Geometry: final body of the model. Coordinates: model frame, mm. Face numbers are marked on the shaded views. A direction names the side the tool comes from. Round coordinates to 2 decimals unless told otherwise and drop trailing zeros. Write each loop counter-clockwise with the first axis right and the second up, starting at its lowest first coordinate (ties: lowest second). Pieces come first, ordered by that corner, then holes. Notation, with made-up numbers: (81, -37.75) -> (129, -37.75) arc R32 ccw to (129, 1.25) -> close; hole circle Ø4 at (-12.75, 67). An arc over 180 degrees is marked (long way). Use one line per item in the form item = value. Start each with the question number.
1. Cut plane B-B, the plane x = 0. Return the cut outline in (y, z).
2. Cut plane D-D, the plane y = 21.5. Return the cut outline in (x, z), plus the area to 3 significant figures.
3. Reachability of the marked faces 4 and 5 from +Z, -Z, +X, -X, +Y, -Y: full face, straight path, thin tool, end or side. Return the list, or none.
4. Line query: L1, parallel to Y at x = -14, z = 2.5; L2, parallel to Y at x = -16.5, z = 3.75; L3, parallel to X at y = 1.5, z = 6. Output: solid intervals per line, ascending.
5. Cut plane C-C, the plane y = 15.5. Return the cut outline in (x, z).
6. Draft query along X for the marked faces 1, 2 and 3. Return one class per face: pulls with the +X half, pulls with the -X half, needs draft (parallel to the pull), parting line crosses it, or undercut.
7. Cut plane A-A, the plane z = 1.5. Return the cut outline in (x, y), plus the area to 3 significant figures.
8. Pin query (flat end, axial travel): pin 1 Ø4 at (x, z) = (-0.5, 2) entering from -Y; pin 2 Ø1.7 at (x, z) = (-15.5, 3) entering from +Y; pin 3 Ø1 at (x, y) = (-18.5, 6.5) entering from +Z; pin 4 Ø4 at (x, y) = (10, -17) entering from -Z. Return the tip coordinate at first contact, or that it passes through.
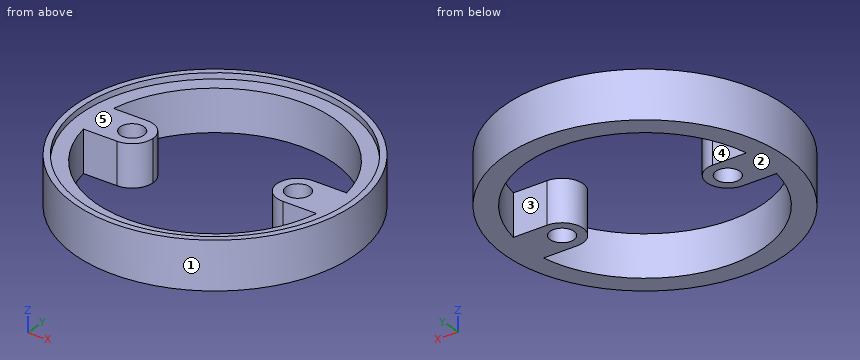
```python
from build123d import *

# Parameters (mm, degrees)
F0_R     = 22.5
F1_DEPTH = 7
F0_R_2   = 23.5
F2_DEPTH = 8
F3_D     = 4


with BuildPart() as f1:
    # F0 (on Top) → F1 (new body)
    with BuildSketch(Plane.XY):
        Circle(F0_R)
        with BuildLine():
            ThreePointArc((19.691369, 3.5), (19.922693, 1.756791), (20, 0))
            ThreePointArc((20, 0), (19.922693, -1.756791), (19.691369, -3.5))
            ThreePointArc((19.691369, -3.5), (0, -20), (-19.691369, -3.5))
            ThreePointArc((-19.691369, -3.5), (-20, 0), (-19.691369, 3.5))
            ThreePointArc((-19.691369, 3.5), (0, 20), (19.691369, 3.5))
        make_face(mode=Mode.SUBTRACT)
        with BuildLine():
            Line((-14, 3.5), (-19.691369, 3.5))
            ThreePointArc((-19.691369, 3.5), (-20, 0), (-19.691369, -3.5))
            Line((-19.691369, -3.5), (-14, -3.5))
            ThreePointArc((-14, -3.5), (-17.5, 0), (-14, 3.5))
        make_face()
        with BuildLine():
            ThreePointArc((-10.5, 0), (-11.525126, 2.474874), (-14, 3.5))
            ThreePointArc((-14, 3.5), (-17.5, 0), (-14, -3.5))
            ThreePointArc((-14, -3.5), (-11.525126, -2.474874), (-10.5, 0))
        make_face()
        with BuildLine():
            ThreePointArc((17.5, 0), (16.474874, 2.474874), (14, 3.5))
            ThreePointArc((14, 3.5), (10.5, 0), (14, -3.5))
            ThreePointArc((14, -3.5), (16.474874, -2.474874), (17.5, 0))
        make_face()
        with BuildLine():
            ThreePointArc((19.691369, -3.5), (19.922693, -1.756791), (20, 0))
            ThreePointArc((20, 0), (19.922693, 1.756791), (19.691369, 3.5))
            Line((19.691369, 3.5), (14, 3.5))
            ThreePointArc((14, 3.5), (16.474874, 2.474874), (17.5, 0))
            ThreePointArc((17.5, 0), (16.474874, -2.474874), (14, -3.5))
            Line((14, -3.5), (19.691369, -3.5))
        make_face()
    extrude(amount=F1_DEPTH)

    # F0 (on Top) → F2 (join)
    with BuildSketch(Plane.XY):
        Circle(F0_R_2)
        Circle(F0_R, mode=Mode.SUBTRACT)
    extrude(amount=F2_DEPTH)

    # F3 (through all)
    with Locations(Plane(origin=(0, 0, 0), x_dir=(1, 0, 0), z_dir=(0, 0, -1))):
        with Locations((-14, 0), (14, 0)):
            Hole(F3_D / 2)


solid = f1.part
```
Outcome:
q1.outline = (-23.5, 0) -> (-20, 0) -> (-20, 7) -> (-22.5, 7) -> (-22.5, 8) -> (-23.5, 8) -> close; (20, 0) -> (23.5, 0) -> (23.5, 8) -> (22.5, 8) -> (22.5, 7) -> (20, 7) -> close
q2.outline = (-9.49, 0) -> (9.49, 0) -> (9.49, 8) -> (6.63, 8) -> (6.63, 7) -> (-6.63, 7) -> (-6.63, 8) -> (-9.49, 8) -> close
q2.area = 139 mm^2
q3.face_4 = +Z, -Z
q3.face_5 = +Z
q4.L1 = -18.87 to -14.28, -3.5 to -2, 2 to 3.5, 14.28 to 18.87
q4.L2 = -16.73 to -11.3, -3.5 to 3.5, 11.3 to 16.73
q4.L3 = -23.45 to -15.32, -12.68 to -10.84, 10.84 to 12.68, 15.32 to 23.45
q5.outline = (-17.66, 0) -> (-12.64, 0) -> (-12.64, 7) -> (-16.31, 7) -> (-16.31, 8) -> (-17.66, 8) -> close; (12.64, 0) -> (17.66, 0) -> (17.66, 8) -> (16.31, 8) -> (16.31, 7) -> (12.64, 7) -> close
q6.face_1 = parting line crosses it
q6.face_2 = needs draft
q6.face_3 = undercut
q7.outline = circle Ø47 at (0, 0); hole (-19.69, -3.5) arc R20 ccw to (19.69, -3.5) -> (14, -3.5) arc R3.5 cw to (14, 3.5) -> (19.69, 3.5) arc R20 ccw to (-19.69, 3.5) -> (-14, 3.5) arc R3.5 cw to (-10.5, 0) arc R3.5 cw to (-14, -3.5) -> close; hole circle Ø4 at (-14, 0); hole circle Ø4 at (14, 0)
q7.area = 574 mm^2
q8.pin_1 = -23.5
q8.pin_2 = 18.37
q8.pin_3 = 7
q8.pin_4 = 0
